Input: part model. Units: mm. Frame: model coordinates. A direction names the side the tool comes from. Round coordinates to 2 decimals unless told otherwise and drop trailing zeros. Write each loop counter-clockwise with the first axis right and the second up, starting at its lowest first coordinate (ties: lowest second). Pieces come first, ordered by that corner, then holes. Notation, with made-up numbers: (-12, 42) -> (46, 42) arc R31 cw to (46, 74) -> close; hole circle Ø8 at (45.5, 6.5). An arc over 180 degrees is marked (long way). Use CSV: the item, a comma, the result in double quotes.
Autodesk Inventor part; units mm, degrees
ref_plane "YZ Plane" through (0, 0, 0) normal (1, 0, 0) x (0, 1, 0)
ref_plane "XZ Plane" through (0, 0, 0) normal (0, 1, 0) x (-1, 0, 0)
ref_plane "XY Plane" through (0, 0, 0) normal (0, 0, 1) x (1, 0, 0)
sketch "Sketch1" plane through (0, 0, 0) normal (0, 0, 1) x (1, 0, 0)
  line L0 (-6.3366, 6.9163) -> (21.6034, 6.9163)
  line L1 (21.6034, 6.9163) -> (21.6034, -8.3237)
  line L2 (21.6034, -8.3237) -> (-6.3366, -8.3237)
  line L3 (-6.3366, -8.3237) -> (-6.3366, 6.9163)
  point P0 (0, 0)
  dimension "d0" = 27.94
  dimension "d1" = 15.24
extrude "Extrusion1" add sketch "Sketch1" along normal blind 7.62
sketch "Sketch2" plane through (0, 0, 7.62) normal (0, 0, 1) x (1, 0, 0)
  line L0 (-6.3366, 6.9163) -> (-6.3366, -8.3237)
  line L1 (21.6034, -8.3237) -> (21.6034, 6.9163)
  line L2 (21.6034, -0.052) -> (21.6034, 2.361)
  line L3 (-6.3366, 2.361) -> (-6.3366, -0.052)
  line L4 (21.6034, 6.9163) -> (-6.3366, 6.9163)
  line L5 (-6.3366, -8.3237) -> (21.6034, -8.3237)
  line L6 (0.9631, 2.361) -> (-0.2406, 2.361)
  line L7 (-0.2406, -0.052) -> (0.9631, -0.052)
  line L8 (-0.2406, -0.052) -> (-0.2406, 2.361)
  line L9 (-0.2406, -0.052) -> (3.0821, -0.052)
  line L10 (3.0821, -0.052) -> (3.0821, 2.361)
  line L11 (3.0821, 2.361) -> (-0.2406, 2.361)
  line L12 (-0.2406, 2.361) -> (-0.2406, -0.052)
  line L13 (14.3038, 2.361) -> (15.5074, 2.361)
  line L14 (15.5074, -0.052) -> (14.3038, -0.052)
  line L15 (15.5074, -0.052) -> (15.5074, 2.361)
  line L16 (15.5074, -0.052) -> (12.1847, -0.052)
  line L17 (12.1847, -0.052) -> (12.1847, 2.361)
  line L18 (12.1847, 2.361) -> (15.5074, 2.361)
  line L19 (15.5074, 2.361) -> (15.5074, -0.052)
  line L20 (-6.3366, -0.7037) -> (21.6034, -0.7037)
  line L21 (-6.3366, 2.361) -> (21.6034, 2.361)
  line L22 (21.6034, 2.361) -> (21.6034, -0.052)
  line L23 (21.6034, -0.052) -> (-6.3366, -0.052)
  line L24 (-6.3366, -0.052) -> (-6.3366, 2.361)
  point P0 (0, 0)
  point P1 (-0.2406, 1.1545)
  point P2 (15.2669, -0.3643)
  point P3 (15.5074, 1.1545)
  point P4 (15.5074, -0.052)
  point P5 (21.6034, -0.052)
  point P6 (15.5074, 2.361)
  point P7 (-6.3366, -0.052)
  point P8 (-0.2406, -0.052)
  point P9 (-0.2406, 2.361)
  point P10 (-6.3366, 2.361)
  point P11 (3.0821, -0.052)
  point P12 (12.1847, -0.052)
  point P13 (12.1847, 2.361)
  point P14 (3.0821, 2.361)
  dimension "d6" = 6.096
extrude "Extrusion2" add sketch "Sketch2" along normal blind 8.7376 contours L6 L11 L10 L9 L7 L8 | L15 L14 L16 L17 L18 L13
sketch "Sketch3" plane through (-0.2406, 2.361, 7.62) normal (0, 1, 0) x (1, 0, 0)
  line L0 (3.3227, -8.7376) -> (0, -8.7376)
  line L1 (-6.096, 7.62) -> (21.844, 7.62)
  line L2 (3.3227, -11.3552) -> (3.3227, -8.7376)
  line L3 (12.4253, -11.3552) -> (12.4253, -8.7376)
  line L4 (17.2091, -8.255) -> (17.2091, -15.2732)
  line L5 (17.2091, -15.2732) -> (14.9854, -19.057)
  line L6 (14.9854, -19.057) -> (12.4253, -19.057)
  line L7 (12.4253, -19.057) -> (12.4253, -8.7376)
  line L8 (7.874, 7.62) -> (7.874, -24.8322)
  line L9 (3.3227, -11.3552) -> (3.3227, -8.7376)
  line L10 (-1.4611, -8.255) -> (-1.4611, -15.2732)
  line L11 (-1.4611, -15.2732) -> (0.7626, -19.057)
  line L12 (0.7626, -19.057) -> (3.3227, -19.057)
  line L13 (3.3227, -19.057) -> (3.3227, -8.7376)
  line L14 (17.2091, -8.255) -> (12.4253, -8.255)
  line L15 (12.4253, 0) -> (12.4253, -8.7376)
  line L16 (12.4253, -8.255) -> (12.4253, -8.7376)
  line L17 (-1.4611, -8.255) -> (3.3227, -8.255)
  line L18 (3.3227, 0) -> (3.3227, -8.7376)
  line L19 (3.3227, -8.255) -> (3.3227, -8.7376)
  point P0 (0.2406, 7.62)
extrude "Extrusion4" add sketch "Sketch2" along normal blind 25.4 contours L6 L11 L10 L9 L7 L8 | L15 L14 L16 L17 L18 L13
sketch "Sketch4" plane through (-6.3366, 6.9163, 0) normal (0, 1, 0) x (1, 0, 0)
  point P0 (6.3366, 0)
sketch "Sketch5" plane through (0, 0, 7.62) normal (0, 0, 1) x (1, 0, 0)
  line L0 (21.6034, 6.9163) -> (-6.3366, 6.9163)
  line L1 (-6.3366, 15.6735) -> (21.6034, 15.6735)
  line L2 (21.6034, 15.6735) -> (21.6034, 6.9163)
  line L3 (21.6034, 6.9163) -> (-6.3366, 6.9163)
  line L4 (-6.3366, 6.9163) -> (-6.3366, 15.6735)
  point P0 (0, 0)
extrude "Extrusion5" add sketch "Sketch5" along normal blind 17.145 and the other way blind 7.62
extrude "Extrusion6" cut sketch "Sketch2" against normal blind 25.4 contours L20 L1 L5 L0
extrude "Extrusion7" add sketch "Sketch2" along normal blind 4.7625 contours L21 L8 L23 L0 | L1 L23 L15 L21 | L21 L17 L23 L10
extrude "Extrusion8" add sketch "Sketch3" against normal up to surface (2.413 mm away)
sketch "Sketch6" plane through (-6.3366, -0.052, 7.62) normal (0, -1, 0) x (1, 0, 0)
  line L0 (27.94, 0) -> (27.94, 4.7625)
  line L1 (21.844, 4.7625) -> (21.844, 8.255)
  line L2 (27.94, 0) -> (21.844, 0)
  line L3 (21.844, 0) -> (21.844, 4.7625)
  line L4 (21.844, 4.7625) -> (27.94, 4.7625)
  line L5 (27.94, 4.7625) -> (27.94, 0)
  line L6 (18.5213, 4.7625) -> (18.5213, 25.4)
  line L7 (18.5213, 4.7625) -> (9.4187, 4.7625)
  line L8 (9.4187, 4.7625) -> (9.4187, 0)
  line L9 (9.4187, 0) -> (18.5213, 0)
  line L10 (18.5213, 0) -> (18.5213, 4.7625)
  line L11 (6.096, 4.7625) -> (6.096, 8.255)
  line L12 (0, 0) -> (0, 4.7625)
  line L13 (6.096, 4.7625) -> (0, 4.7625)
  line L14 (0, 4.7625) -> (0, 0)
  line L15 (0, 0) -> (6.096, 0)
  line L16 (6.096, 0) -> (6.096, 4.7625)
  point P0 (6.3366, -7.62)
  point P1 (21.844, 8.7376)
  point P2 (18.5213, 19.057)
  point P3 (6.096, 8.7376)
extrude "Extrusion9" cut sketch "Sketch6" against normal up to surface (6.9683 mm away)
sketch "Sketch7" plane through (12.1847, -0.052, 7.62) normal (0, -1, 0) x (1, 0, 0)
  line L0 (3.3227, 17.7594) -> (4.7838, 15.2732)
  line L1 (3.3227, 17.7594) -> (2.3659, 19.3874)
  line L2 (2.3659, 19.3874) -> (2.3659, 25.4)
  line L3 (3.3227, 25.4) -> (0, 25.4)
  line L4 (3.3227, 17.7594) -> (3.3227, 25.4)
  line L5 (2.3659, 25.4) -> (3.3227, 25.4)
  line L6 (3.3227, 25.4) -> (3.3227, 17.7594)
  line L7 (-18.5213, -7.62) -> (9.4187, -7.62)
  line L8 (-12.4253, 17.7594) -> (-11.4685, 19.3874)
  line L9 (-11.4685, 19.3874) -> (-11.4685, 25.4)
  line L10 (-12.4253, 17.7594) -> (-12.4253, 25.4)
  line L11 (-11.4685, 25.4) -> (-12.4253, 25.4)
  line L12 (-12.4253, 25.4) -> (-12.4253, 17.7594)
  line L13 (-12.4253, 8.7376) -> (-13.8865, 8.255)
  line L14 (-9.1825, 8.7376) -> (-9.1026, 8.7376)
  line L15 (-9.1026, 0) -> (-9.1026, 25.4)
  line L16 (-10.6842, 5.3569) -> (-10.764, 0)
  line L17 (-9.1026, 0) -> (-12.4253, 0)
  line L18 (-9.1026, 0) -> (-9.1026, 8.7376)
  line L19 (-10.764, 0) -> (-9.1026, 0)
  line L20 (9.4187, -7.62) -> (-18.5213, -7.62)
  line L21 (-18.5213, 17.145) -> (9.4187, 17.145)
  line L22 (1.5816, 5.3569) -> (1.6613, 0)
  line L23 (1.6613, 0) -> (0, 0)
  line L24 (0, 0) -> (0, 8.7376)
  line L25 (-4.5513, -7.62) -> (-4.5513, 0)
  line L26 (-4.5513, 11.274) -> (-4.5513, 11.3382)
  line L27 (-9.1026, 8.7376) -> (-10.6842, 5.3569)
  line L28 (0, 8.7376) -> (1.5816, 5.3569)
  point P0 (-12.1847, -7.62)
extrude "Extrusion10" cut sketch "Sketch7" against normal up to surface (6.9683 mm away)
fillet "Fillet1" radius 3.175 4 edges at (0.7162, 1.1545, 33.02) (14.5507, 1.1545, 33.02) (16.9686, 1.1545, 22.8932) (-1.7017, 1.1545, 22.8932)
sketch "Sketch8" plane through (-0.2406, -0.052, 7.62) normal (0, -1, 0) x (1, 0, 0)
  arc A0 (-1.0234, 16.018) -> (-1.4611, 14.4093) centre (1.7139, 14.4093) ccw
  line L0 (-1.4611, 8.255) -> (-1.4611, 14.4093)
  line L1 (0, 0) -> (0, 8.255)
  line L2 (1.6613, 0) -> (0, 0)
  line L3 (1.6613, 0) -> (1.7411, 5.3569)
  line L4 (1.7411, 5.3569) -> (3.3227, 8.7376)
  line L5 (3.3227, 8.7376) -> (3.3227, 25.4)
  arc A1 (3.3227, 25.4) -> (0.9568, 22.3298) centre (4.1318, 22.3298) ccw
  line L6 (0.9568, 22.3298) -> (0.9568, 19.3874)
  line L7 (0.9568, 19.3874) -> (-1.0234, 16.018)
  arc A2 (17.2091, 14.4093) -> (16.7714, 16.018) centre (14.0341, 14.4093) ccw
  line L8 (16.7714, 16.018) -> (14.7912, 19.3874)
  line L9 (14.7912, 19.3874) -> (14.7912, 22.3298)
  arc A3 (14.7912, 22.3298) -> (12.4253, 25.4) centre (11.6162, 22.3298) ccw
  line L10 (12.4253, 8.7376) -> (12.4253, 25.4)
  line L11 (12.4253, 8.7376) -> (14.0069, 5.3569)
  line L12 (14.0069, 5.3569) -> (14.0867, 0)
  line L13 (15.748, 0) -> (14.0867, 0)
  line L14 (15.748, 0) -> (15.748, 8.255)
  line L15 (17.2091, 14.4093) -> (17.2091, 8.255)
  line L16 (17.2091, 8.255) -> (15.748, 8.255)
  line L17 (0, 8.255) -> (-1.4611, 8.255)
  point P0 (0.2406, -7.62)
extrude "Extrusion11" add sketch "Sketch8" against normal blind 3.81
sketch "Sketch9" plane through (0, 0, 7.62) normal (0, 0, 1) x (1, 0, 0)
  line L0 (9.6447, 0.3123) -> (5.6221, 0.3123)
  line L1 (5.6221, 0.3123) -> (5.6221, 4.1223)
  line L2 (5.6221, 4.1223) -> (9.6447, 4.1223)
  line L3 (9.6447, 4.1223) -> (9.6447, 0.3123)
  line L4 (12.1847, -0.052) -> (12.1847, 3.758)
  line L5 (3.0821, -0.052) -> (3.0821, 3.758)
  point P0 (0, 0)
  dimension "d30" = 2.54
  dimension "d31" = 2.54
extrude "Extrusion12" add sketch "Sketch9" along normal blind 18.0975
properties part number "Attachment5"
Item 1: Pull-direction query (Z, two-part tool) for faces 6 (the face through (15.507, 2, 12)), 7 (the face through (5.622, 2, 17)), 8 (the face through (8, 2, 25.718)); classes: +Z half, -Z half, draft (parallel to the pull), parting line (faces both ways), or undercut.
Worked answers:
face 6,"undercut"
face 7,"draft"
face 8,"+Z half"
Item 2: Line query: line 1 (Y direction, x = -1, z = 23); line 2 (Z direction, x = 9, y = 10.25) (3 decimals); line 3 (X direction, y = 2.25, z = 25). Output: solid intervals per line, ascending.
Worked answers:
line 1,"y = -0.05 to 3.76, 6.92 to 15.67"
line 2,"z = 0 to 24.765"
line 3,"x = -0.46 to 3.08, 5.62 to 9.64, 12.18 to 15.73"
Item 3: Set-up query: faces 1 (the face through (1, -0.052, 20)), 2 (the face through (2.3, 1.83, 14.69)), 3 (the face through (8, 0.312, 17)), 4 (the face through (-1, 2, 15.875)), 5 (the face through (16.86, 3.05, 22.85)). Return all of +Z, -Z, +X, -X, +Y, -Y with unobstructed straight access to the full face (end or side cutting, diameter ignored); none if empty.
Worked answers:
face 1,"+Z, +X, -X, -Y"
face 2,"-Y"
face 3,"+Z, -Y"
face 4,"-X, -Y"
face 5,"+Z, +X, -Y"
Item 4: Section query C-C on z = 28. Return the cut outline in (x, y), plus the area to 3 significant figures.
Worked answers:
outline,"(0.72, -0.05) -> (3.08, -0.05) -> (3.08, 3.76) -> (0.72, 3.76) -> close; (12.18, -0.05) -> (14.55, -0.05) -> (14.55, 3.76) -> (12.18, 3.76) -> close"
area,"18.0 mm²"
Item 5: First-contact query: pin 1 Ø2.5 at (x, y) = (11.5, 11.5) entering from +Z (3 decimals); pin 2 Ø5 at (x, z) = (14.5, 12) entering from -Y; pin 3 Ø3 at (y, z) = (3, 19.5) entering from -X. Flat tips, straight axial feed; report the tip coordinate or a pass-through.
Worked answers:
pin 1,"stops at z = 24.765"
pin 2,"stops at y = -0.05"
pin 3,"stops at x = -1.7"
Item 6: Section query A-A on z = 19. Return the cut outline in (x, y).
Worked answers:
outline,"(-6.34, 6.92) -> (21.6, 6.92) -> (21.6, 15.67) -> (-6.34, 15.67) -> close; (-1.7, -0.05) -> (3.08, -0.05) -> (3.08, 3.76) -> (-1.7, 3.76) -> close; (5.62, 0.31) -> (9.64, 0.31) -> (9.64, 4.12) -> (5.62, 4.12) -> close; (12.18, -0.05) -> (16.97, -0.05) -> (16.97, 3.76) -> (12.18, 3.76) -> close"
Item 7: Section query D-D on x = 2.5. Return the cut outline in (y, z) (1 decimal).
Worked answers:
outline,"(-0.7, 0) -> (15.7, 0) -> (15.7, 24.8) -> (6.9, 24.8) -> (6.9, 7.6) -> (-0.7, 7.6) -> close; (-0.1, 15.1) -> (3.8, 15.1) -> (3.8, 32.8) -> (-0.1, 32.8) -> close"
